Build history of the part. All positions in model axes, mm. A direction names the side the tool comes from. Give positions to 0.01 mm unless a question says otherwise; leave off trailing zeros. Write each loop counter-clockwise with the first axis right and the second up, starting at its lowest first coordinate (ties: lowest second). Pieces come first, ordered by that corner, then holes.
from build123d import *

# Parameters (mm, degrees)
F0_W     = 50
F0_H     = 50
F1_DEPTH = 50
F2_T     = -2.5
F3_R     = 5


with BuildPart() as f1:
    # F0 (on Top) → F1 (new body)
    with BuildSketch(Plane.XY):
        Rectangle(F0_W, F0_H)
    extrude(amount=F1_DEPTH)

    # F2
    f2_openings = [f1.faces().sort_by_distance(p)[0] for p in [
        (0, 0, 50),
    ]]
    offset(amount=F2_T, openings=f2_openings)

    # F3
    f3_edges = [f1.edges().sort_by_distance(p)[0] for p in [
        (-25, -25, 25),
        (25, -25, 25),
        (25, 25, 25),
        (-25, 25, 25),
    ]]
    fillet(f3_edges, radius=F3_R)


solid = f1.part
1. Drill centre lines: line 1 along Y through (x, z) = (18, 24); line 2 along Z through (x, y) = (-17, -6). Where is each one in solid material? Low to high.
2. Drop flat-ended pins along their axis: pin 1 (3 mm diameter, centred on x = 17.5, y = -10, fed in from -Z); pin 2 (22.5 mm diameter, centred on x = 0.5, y = -1.5, fed in from +Z). Give the stop position or say it passes through.
3. Mould opens along Y. For faces 1 (the face through (22.5, 0, 26)), 2 (the face through (0, 0, 2.5)), 3 (the face through (0, 25, 25)), 4 (the face through (0, 0, 0)) say: pulls with the +Y half, pulls with the -Y half, needs draft (parallel to the pull), parting line crosses it, or undercut.
4. Saw through at A-A on z = 19. Give the cut face in (x, y).
5. 3-axis set-ups, long thin cutter, end or side, ignore diameter. For faces 5 (the face through (0, -22.5, 26)), 6 (the face through (23, -24, 25)): which of +Z, -Z, +X, -X, +Y, -Y reach the whole face in a straight line?
6. Saw through at B-B on x = 6.5. Give the cut face in (y, z), plus the area to 4 significant figures.
Outcome:
1. line 1: y = -25 to -22.5, 22.5 to 25
1. line 2: z = 0 to 2.5
2. pin 1: stops at z = 0
2. pin 2: stops at z = 2.5
3. face 1: undercut
3. face 2: undercut
3. face 3: pulls with the +Y half
3. face 4: needs draft
4. outline: (-25, -20) arc R5 ccw to (-20, -25) - (20, -25) arc R5 ccw to (25, -20) - (25, 20) arc R5 ccw to (20, 25) - (-20, 25) arc R5 ccw to (-25, 20) - close; hole (-22.5, -22.5) - (22.5, -22.5) - (22.5, 22.5) - (-22.5, 22.5) - close
5. face 5: +Z
5. face 6: +Z, -Z, +X, -Y
6. outline: (-25, 0) - (25, 0) - (25, 50) - (22.5, 50) - (22.5, 2.5) - (-22.5, 2.5) - (-22.5, 50) - (-25, 50) - close
6. area: 362.5 mm2
